Verification items for the finished model (mm, model axes). Give positions to 0.01 mm unless a question says otherwise; leave off trailing zeros. Loops run counter-clockwise (first coordinate to the right, second up) from the corner with the lowest first, then second, coordinate; pieces in that order, holes last. Notation, with made-up numbers: (65.25, 57.25) -> (87.25, 57.25) arc R23 cw to (87.25, 65.25) -> close; hole circle Ø3 at (-25.75, 21.25). An arc over 180 degrees is marked (long way). Answer in a Markdown table with one row per item. Add a question column.
Q1. Section check B-B on z = 0.1. Give the number of separate pieces and of enclosed holes in the cut face, and give its area (3 significant figures).
Q2. Section check A-A on y = 104. Enter the section's corners in (x, z), and give its area (3 significant figures).
Q3. Material ranges on probe 1 along X at (y, z) = (-107.5, 0.2); probe 2 along Y at (x, z) = (-16, 0.1); probe 3 along X at (y, z) = (115, 0.15), recorded low to high.
Q4. Section check C-C on x = -72.5. Enter the section's corners in (y, z).
```python
from build123d import *

# Parameters (mm, degrees)
F1_W     = 254
F1_H     = 254
F2_DEPTH = 0.254


with BuildPart() as f2:
    # F1 (on Top) → F2 (new body)
    with BuildSketch(Plane.XY):
        Rectangle(F1_W, F1_H)
        Polygon((-0.254, -126.492), (-126.13279, -126.492), (-0.254, -0.61321), align=None, mode=Mode.SUBTRACT)
        Polygon((-0.61321, -0.254), (-126.492, -126.13279), (-126.492, -0.254), align=None, mode=Mode.SUBTRACT)
        Polygon((126.13279, -126.492), (0.254, -126.492), (0.254, -0.61321), align=None, mode=Mode.SUBTRACT)
        Polygon((126.492, -0.254), (126.492, -126.13279), (0.61321, -0.254), align=None, mode=Mode.SUBTRACT)
        Polygon((-126.492, 0.254), (-126.492, 126.13279), (-0.61321, 0.254), align=None, mode=Mode.SUBTRACT)
        Polygon((-0.254, 0.61321), (-126.13279, 126.492), (-0.254, 126.492), align=None, mode=Mode.SUBTRACT)
        Polygon((0.61321, 0.254), (126.492, 126.13279), (126.492, 0.254), align=None, mode=Mode.SUBTRACT)
        Polygon((0.254, 0.61321), (0.254, 126.492), (126.13279, 126.492), align=None, mode=Mode.SUBTRACT)
    extrude(amount=F2_DEPTH)


solid = f2.part
```
Taken from the geometry:
| question | item | result |
|---|---|---|
| 1 | separate pieces | 1 |
| 1 | enclosed holes | 8 |
| 1 | area | 1,130 mm² |
| 2 | outline | (-127, 0) -> (-126.49, 0) -> (-126.49, 0.25) -> (-127, 0.25) -> close; (-104.36, 0) -> (-103.64, 0) -> (-103.64, 0.25) -> (-104.36, 0.25) -> close; (-0.25, 0) -> (0.25, 0) -> (0.25, 0.25) -> (-0.25, 0.25) -> close; (103.64, 0) -> (104.36, 0) -> (104.36, 0.25) -> (103.64, 0.25) -> close; (126.49, 0) -> (127, 0) -> (127, 0.25) -> (126.49, 0.25) -> close |
| 2 | area | 0.752 mm² |
| 3 | probe 1 | x = -127 to -126.49, -107.86 to -107.14, -0.25 to 0.25, 107.14 to 107.86, 126.49 to 127 |
| 3 | probe 2 | y = -127 to -126.49, -16.36 to -15.64, -0.25 to 0.25, 15.64 to 16.36, 126.49 to 127 |
| 3 | probe 3 | x = -127 to -126.49, -115.36 to -114.64, -0.25 to 0.25, 114.64 to 115.36, 126.49 to 127 |
| 4 | outline | (-127, 0) -> (-126.49, 0) -> (-126.49, 0.25) -> (-127, 0.25) -> close; (-72.86, 0) -> (-72.14, 0) -> (-72.14, 0.25) -> (-72.86, 0.25) -> close; (-0.25, 0) -> (0.25, 0) -> (0.25, 0.25) -> (-0.25, 0.25) -> close; (72.14, 0) -> (72.86, 0) -> (72.86, 0.25) -> (72.14, 0.25) -> close; (126.49, 0) -> (127, 0) -> (127, 0.25) -> (126.49, 0.25) -> close |
